from build123d import *

# Parameters (mm, degrees)
F0_R     = 9.5
F0_R_2   = 2.5
F1_DEPTH = 2.5
F2_R     = 1.5
F3_DEPTH = 5.001
F4_R     = 1.25
F5_DEPTH = 9.501
F6_SIZE  = 0.1


with BuildPart() as f1:
    # F0 (on Right) → F1 (new body, symmetric)
    with BuildSketch(Plane.YZ):
        Circle(F0_R)
        Circle(F0_R_2, mode=Mode.SUBTRACT)
    extrude(amount=F1_DEPTH, both=True)

    # F2 (on face) → F3 (cut, through all)
    with BuildSketch(Plane.YZ.offset(2.5)):
        with Locations((-4.490128, 4.490128)):
            Circle(F2_R)
        with Locations((-4.490128, -4.490128)):
            Circle(F2_R)
        with Locations((4.490128, -4.490128)):
            Circle(F2_R)
        with Locations((4.490128, 4.490128)):
            Circle(F2_R)
    extrude(amount=-F3_DEPTH, mode=Mode.SUBTRACT)

    # F4 (on Front) → F5 (cut, through all)
    with BuildSketch(Plane.XZ):
        Circle(F4_R)
    extrude(amount=F5_DEPTH, mode=Mode.SUBTRACT)

    # F6
    f6_edges = [f1.edges().sort_by_distance(p)[0] for p in [
        (2.5, -9.5, 0),
        (2.5, -5.990128, -4.490128),
        (2.5, 2.990128, -4.490128),
        (2.5, -5.990128, 4.490128),
        (2.5, -2.5, 0),
        (2.5, 2.990128, 4.490128),
        (-2.5, -9.5, 0),
        (-2.5, -5.990128, -4.490128),
        (-2.5, 2.990128, -4.490128),
        (-2.5, -5.990128, 4.490128),
        (-2.5, -2.5, 0),
        (-2.5, 2.990128, 4.490128),
    ]]
    chamfer(f6_edges, length=F6_SIZE)


solid = f1.part
Read the model definition and answer for the solid it produces. Units are mm, in the model's axes. A direction names the side the tool comes from. Give positions to 0.01 mm unless a question says otherwise; leave off trailing zeros. Write each loop counter-clockwise with the first axis right and the second up, starting at its lowest first coordinate (ties: lowest second). Pieces come first, ordered by that corner, then holes. Notation, with made-up numbers: (18, 69) - (77, 69) arc R13 cw to (77, 77) - close; hole circle Ø3 at (56, 71.5). An arc over 180 degrees is marked (long way). Use CSV: the item, a comma, the result in double quotes. Start each with the question number.
(1) Consider line 1 along Y through (x, z) = (-2.05, 4.25); line 2 along Y through (x, z) = (-1.4, 5.5); line 3 along Z through (x, y) = (0.25, -7.25). Determine where each line is inside the solid, lowest interval first.
(2) Find section B-B (y = 0). Give the vertices of the cut face in (x, z), plus the area to 3 significant figures.
(3) Given P1, Ø1.5, axis at x = -1, y = -6, coming from the +Z side; P2, Ø2, axis at x = 0, z = -5, coming from the -Y side; P3, Ø2, axis at x = 0, z = 6, coming from the +Y side; P4, Ø1.8, axis at y = -4.49, z = 4.49, coming from the +X side, each flat-ended and moving along its own axis, determine where each tip first touches the part or whether it passes through.
(4) For faces 4 (the cylindrical face through (-0.27, -5.78, -1.22)), 5 (the cylindrical face through (0.034, 5.876, 3.916)), determine the directions among +Z, -Z, +X, -X, +Y, -Y from which every point of the face is accessible in a straight line to the end or side of a thin tool.
(5) Find section A-A (z = 0). Give the vertices of the cut face in (x, y).
(6) Determine the mould class of faces 1 (the cylindrical face through (0.034, 9.061, 2.854)), 2 (the flat face through (2.5, 2, -2)), 3 (the cylindrical face through (-0.03, 2.31, -0.96)) for opening direction Z: +Z half, -Z half, draft (parallel to the pull), parting line (faces both ways), or undercut.
(7) Find section D-D (y = -3.75). Count the separate pieces of the cut face and the enclosed holes in it, plus the area to 3 significant figures.
(8) Find section C-C (x = -1). Give the vertices of the cut face in (y, z).
Findings below:
1,line 1,"-8.5 to -5.97, -3.01 to 3.01, 5.97 to 8.5"
1,line 2,"-7.75 to -5.6, -3.38 to 3.38, 5.6 to 7.75"
1,line 3,"-6.14 to -1.22, 1.22 to 6.14"
2,outline,"(-2.5, -9.4) - (-2.4, -9.5) - (2.4, -9.5) - (2.5, -9.4) - (2.5, -2.6) - (2.4, -2.5) - (-2.4, -2.5) - (-2.5, -2.6) - close; (-2.5, 2.6) - (-2.4, 2.5) - (2.4, 2.5) - (2.5, 2.6) - (2.5, 9.4) - (2.4, 9.5) - (-2.4, 9.5) - (-2.5, 9.4) - close"
2,area,"70.0 mm2"
3,P1,"z = 7.92"
3,P2,"y = -8.62"
3,P3,"y = 8.08"
3,P4,"through"
4,face 4,"-Y"
4,face 5,"+X, -X"
5,outline,"(-2.5, -9.4) - (-2.4, -9.5) - (-1.25, -9.5) - (-1.25, -2.5) - (-2.4, -2.5) - (-2.5, -2.6) - close; (-2.5, 2.6) - (-2.4, 2.5) - (2.4, 2.5) - (2.5, 2.6) - (2.5, 9.4) - (2.4, 9.5) - (-2.4, 9.5) - (-2.5, 9.4) - close; (1.25, -9.5) - (2.4, -9.5) - (2.5, -9.4) - (2.5, -2.6) - (2.4, -2.5) - (1.25, -2.5) - close"
6,face 1,"parting line"
6,face 2,"draft"
6,face 3,"undercut"
7,separate pieces,"3"
7,enclosed holes,"1"
7,area,"56.2 mm2"
8,outline,"(-9.47, -0.75) arc R9.5 ccw (long way) to (-9.47, 0.75) - (-2.38, 0.75) arc R2.5 cw (long way) to (-2.38, -0.75) - close; hole circle Ø3 at (-4.49, -4.49); hole circle Ø3 at (-4.49, 4.49); hole circle Ø3 at (4.49, -4.49); hole circle Ø3 at (4.49, 4.49)"
